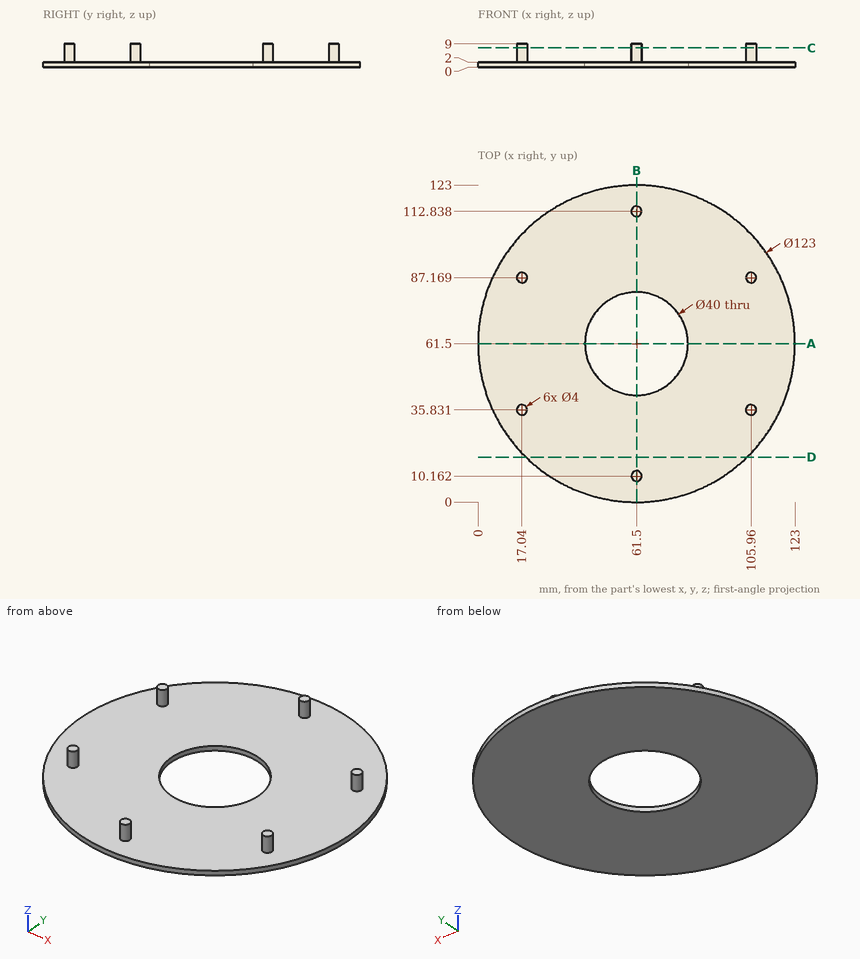
Can you work these out from the drawing? Everything is in mm from the part's minimum corner. Give positions to 0.01 mm unless a question says otherwise; leave off trailing zeros. Order: outer loops, then holes, each group sorted by start corner. A loop starts at its lowest first (then second) coordinate and runs counter-clockwise, first axis right, second up. Notation, with made-up numbers: M 57.5,27.25 L 76.5,27.25 A28 ccw 76.5,55.25 Z; hole C 7,36.5 d10. An arc over 180 degrees is marked long. Use a Markdown table: item, result. Add a question column.
1. Suppose I cut it at B-B (x = 61.5). List the corners of the cut face in (y, z) for me, and give its area (3 significant figures).
2. Suppose I cut it at D-D (y = 17.5). List the corners of the cut face in (x, z) for me, and give its area (3 significant figures).
3. Suppose I cut it at A-A (y = 61.5). List the corners of the cut face in (x, z) for me, and give its area (3 significant figures).
4. Suppose I cut it at C-C (z = 7.5). List the corners of the cut face in (x, y) for me.
5. I need wall thicknesses on probe 1 along Y at (x, z) = (61.5, 1.15); probe 2 along Z at (x, y) = (45, 37.5); probe 3 along Y at (x, z) = (107.5, 5.75) (1 decimal). Which ranges of each line are inside material? Lowest first, please. Write a range as from..to.
6. For pin 1 Ø5 at (x, z) = (66.5, 5.5) entering from +Y; pin 2 Ø4 at (y, z) = (91.5, 1) entering from -X; pin 3 Ø8 at (x, y) = (47, 81) entering from +Z, each with a flat end and sliding along its axis, tell me the tip position at first contact or that it passes through.
Results list:
| question | item | result |
|---|---|---|
| 1 | outline | M 0,0 L 41.5,0 L 41.5,2 L 12.16,2 L 12.16,9 L 8.16,9 L 8.16,2 L 0,2 Z; M 81.5,0 L 123,0 L 123,2 L 114.84,2 L 114.84,9 L 110.84,9 L 110.84,2 L 81.5,2 Z |
| 1 | area | 222 mm² |
| 2 | outline | M 18.53,0 L 104.47,0 L 104.47,2 L 18.53,2 Z |
| 2 | area | 172 mm² |
| 3 | outline | M 0,0 L 41.5,0 L 41.5,2 L 0,2 Z; M 81.5,0 L 123,0 L 123,2 L 81.5,2 Z |
| 3 | area | 166 mm² |
| 4 | outline | C 17.04,35.83 d4; C 17.04,87.17 d4; C 61.5,10.16 d4; C 61.5,112.84 d4; C 105.96,35.83 d4; C 105.96,87.17 d4 |
| 5 | probe 1 | y = 0..41.5, 81.5..123 |
| 5 | probe 2 | z = 0..2 |
| 5 | probe 3 | y = 34.6..37.1, 85.9..88.4 |
| 6 | pin 1 | passes through |
| 6 | pin 2 | stops at x = 6.74 |
| 6 | pin 3 | stops at z = 2 |
